```python
from build123d import *

# Parameters (mm, degrees)
MODEL_R             = 3.96545
MODEL_W             = 1.574799418
MODEL_H             = 12.699998915
MODEL_W_2           = 5.587999709
MODEL_H_2           = 15.087600797
MODEL_W_3           = 7.66
MODEL_H_3           = 10.87
BOSS_EXTRUDE1_DEPTH = 3.048


with BuildPart() as part:
    # Model → Boss-Extrude1 (new body)
    with BuildSketch(Plane.XY):
        with BuildLine():
            Line((25.653999648, 91.084402986), (15.189199708, 91.084402986))
            Line((15.189199708, 91.084402986), (15.189199708, 88.011001237))
            Line((15.189199708, 88.011001237), (25.653999648, 88.011001237))
            Line((25.653999648, 88.011001237), (25.653999648, 81.675999849))
            Line((25.653999648, 81.675999849), (28.323999648, 81.675999849))
            Line((28.323999648, 81.675999849), (30.823999648, 79.175999849))
            Line((30.823999648, 79.175999849), (30.823999648, 53.369499849))
            ThreePointArc((30.823999648, 53.369499849), (30.38465982, 52.308839677), (29.323999648, 51.869499849))
            Line((29.323999648, 51.869499849), (25.653999648, 51.869499849))
            Line((25.653999648, 51.869499849), (25.653999648, 39.189499849))
            Line((25.653999648, 39.189499849), (29.323999648, 39.189499849))
            ThreePointArc((29.323999648, 39.189499849), (30.38465982, 38.750160021), (30.823999648, 37.689499849))
            Line((30.823999648, 37.689499849), (30.823999648, 11.882999849))
            Line((30.823999648, 11.882999849), (28.323999648, 9.382999849))
            Line((28.323999648, 9.382999849), (25.653999648, 9.382999849))
            Line((25.653999648, 9.382999849), (25.653999648, 0))
            Line((25.653999648, 0), (17.399000004, 0))
            Line((17.399000004, 0), (17.399000004, 3.047999926))
            Line((17.399000004, 3.047999926), (11.099800467, 3.047999926))
            Line((11.099800467, 3.047999926), (11.099800467, 0))
            Line((11.099800467, 0), (3.174999729, 0))
            Line((3.174999729, 0), (3.174999729, 9.397999849))
            Line((3.174999729, 9.397999849), (0, 9.397999849))
            Line((0, 9.397999849), (0, 56.261000223))
            Line((0, 56.261000223), (3.174999729, 56.261000223))
            Line((3.174999729, 56.261000223), (3.174999729, 67.817998119))
            Line((3.174999729, 67.817998119), (0, 67.817998119))
            Line((0, 67.817998119), (0, 97.180393524))
            Line((0, 97.180393524), (25.653999648, 97.180393524))
            Line((25.653999648, 97.180393524), (25.653999648, 91.084402986))
        make_face()
        with Locations((18.027649688, 56.534049926)):
            Circle(MODEL_R, mode=Mode.SUBTRACT)
        with Locations((3.657599911, 81.661001779)):
            Rectangle(MODEL_W, MODEL_H, mode=Mode.SUBTRACT)
        with Locations((17.487899866, 34.848800861)):
            Rectangle(MODEL_W_2, MODEL_H_2, mode=Mode.SUBTRACT)
        with Locations((19.907249836, 13.696949929)):
            Rectangle(MODEL_W_3, MODEL_H_3, mode=Mode.SUBTRACT)
    extrude(amount=BOSS_EXTRUDE1_DEPTH)


solid = part.part
```
Geometry check sheet. Reference: the model listing, model coordinates, mm. A direction names the side the tool comes from. Give positions to 0.01 mm unless a question says otherwise; leave off trailing zeros. Order: outer loops, then holes, each group sorted by start corner. A loop starts at its lowest first (then second) coordinate and runs counter-clockwise, first axis right, second up.
1. Access from +Z, -Z, +X, -X, +Y, -Y to the whole of each face (thin tool, end or side, straight path). Record for faces 4 (the face through (14, 3.048, 2)), 5 (the face through (27, 39.189, 2)), 6 (the face through (3.175, 62, 2)), 7 (the face through (3.175, 5, 2)), 8 (the face through (20, 19.132, 2)).
2. Section check B-B, the plane x = 12. Enter the section's corners in (y, z), and give its area (3 significant figures).
3. Thickness scan on L1, parallel to Y at x = 18, z = 2.2 (3 decimals); L2, parallel to X at y = 40, z = 1.7; L3, parallel to X at y = 87.5, z = 0.9 (3 decimals). Record the ranges inside material, lowest first.
4. Section check A-A, the plane y = 33. Enter the section's corners in (x, z).
5. Gauge pin test, flat ends, axial feed: pin 1 Ø1.5 at (x, z) = (1, 1) entering from -Y; pin 2 Ø1.5 at (y, z) = (3.5, 1) entering from +X; pin 3 Ø1.5 at (x, z) = (13, 1.5) entering from -Y. Record the tip position at first contact, or that the pin passes through.
6. Section check C-C, the plane y = 49. Enter the section's corners in (x, z).
7. Release check for a two-part mould opening along Y. For faces 1 (the face through (17.168, 52.663, 1.503)), 2 (the face through (25.654, 5, 2)), 3 (the face through (27, 81.676, 2)) record: pulls with the +Y half, pulls with the -Y half, needs draft (parallel to the pull), parting line crosses it, or undercut.
8. Section check D-D, the plane z = 1.85. Give the number of separate pieces and of enclosed holes in the cut face, and give its area (3 significant figures).
Values follow:
1. face 4: +Z, -Z, -Y
1. face 5: +Z, -Z, +X
1. face 6: +Z, -Z, -X
1. face 7: +Z, -Z, -X, -Y
1. face 8: +Z, -Z
2. outline: (3.05, 0) - (97.18, 0) - (97.18, 3.05) - (3.05, 3.05) - close
2. area: 287 mm2
3. L1: y = 0 to 8.262, 19.132 to 27.305, 42.393 to 52.569, 60.499 to 88.011, 91.084 to 97.18
3. L2: x = 0 to 14.69, 20.28 to 25.65
3. L3: x = 0 to 2.87, 4.445 to 25.654
4. outline: (0, 0) - (14.69, 0) - (14.69, 3.05) - (0, 3.05) - close; (20.28, 0) - (30.82, 0) - (30.82, 3.05) - (20.28, 3.05) - close
5. pin 1: stops at y = 9.4
5. pin 2: stops at x = 25.65
5. pin 3: stops at y = 3.05
6. outline: (0, 0) - (25.65, 0) - (25.65, 3.05) - (0, 3.05) - close
7. face 1: undercut
7. face 2: needs draft
7. face 3: pulls with the +Y half
8. separate pieces: 1
8. enclosed holes: 4
8. area: 2,440 mm2
